from build123d import *

# Parameters (mm, degrees)
SK_PLATE_W              = 160
SK_PLATE_H              = 40
EX_PLATE_DEPTH          = 5
SK_PADPOCKETS_W         = 26
SK_PADPOCKETS_H         = 20
CUT_PADPOCKETS_DEPTH    = 1
SK_PADINSERTS_M3_R      = 2
CUT_PADINSERTS_M3_DEPTH = 5
SK_MAGNET_R             = 3
CUT_MAGNET_DEPTH        = 3
SK_FRAMEBOLTS_R         = 2.15
CUT_FRAMEBOLTS_DEPTH    = 5


with BuildPart() as part:
    # SK_Plate → EX_Plate (new body)
    with BuildSketch(Plane(origin=(0, 0, 0), x_dir=(1, 0, 0), z_dir=(0, 1, 0))):
        Rectangle(SK_PLATE_W, SK_PLATE_H)
    extrude(amount=EX_PLATE_DEPTH)

    # SK_PadPockets → CUT_PadPockets (cut)
    with BuildSketch(Plane(origin=(0, 0, 0), x_dir=(1, 0, 0), z_dir=(0, 1, 0))):
        with Locations((64, 0)):
            Rectangle(SK_PADPOCKETS_W, SK_PADPOCKETS_H)
        with Locations((-64, 0)):
            Rectangle(SK_PADPOCKETS_W, SK_PADPOCKETS_H)
    extrude(amount=CUT_PADPOCKETS_DEPTH, mode=Mode.SUBTRACT)

    # SK_PadInserts_M3 → CUT_PadInserts_M3 (cut)
    with BuildSketch(Plane(origin=(0, 0, 0), x_dir=(1, 0, 0), z_dir=(0, 1, 0))):
        with Locations(Location((64, 0, 0), (0, 0, 270))):
            Circle(SK_PADINSERTS_M3_R)
        with Locations(Location((-64, 0, 0), (0, 0, 270))):
            Circle(SK_PADINSERTS_M3_R)
    extrude(amount=CUT_PADINSERTS_M3_DEPTH, mode=Mode.SUBTRACT)

    # SK_Magnet → CUT_Magnet (cut)
    with BuildSketch(Plane(origin=(0, 0, 0), x_dir=(1, 0, 0), z_dir=(0, 1, 0))):
        with Locations(Location((0, 0, 0), (0, 0, 270))):
            Circle(SK_MAGNET_R)
    extrude(amount=CUT_MAGNET_DEPTH, mode=Mode.SUBTRACT)

    # SK_FrameBolts → CUT_FrameBolts (cut)
    with BuildSketch(Plane(origin=(0, 0, 0), x_dir=(1, 0, 0), z_dir=(0, 1, 0))):
        with Locations(Location((60, 14, 0), (0, 0, 270))):
            Circle(SK_FRAMEBOLTS_R)
        with Locations(Location((-60, 14, 0), (0, 0, 270))):
            Circle(SK_FRAMEBOLTS_R)
    extrude(amount=CUT_FRAMEBOLTS_DEPTH, mode=Mode.SUBTRACT)


solid = part.part
Work out the finished part from the listing and answer in its coordinate system (mm). A direction names the side the tool comes from. Coordinates: 2 decimals unless noted, no trailing zeros. Loops run counter-clockwise (first coordinate to the right, second up) from the corner with the lowest first, then second, coordinate; pieces in that order, holes last. Notation, with made-up numbers: M 0.5,-3.75 L 9.5,-3.75 A26 cw 9.5,11.25 Z; hole C 25.5,80 d11. An arc over 180 degrees is marked long. Answer in a Markdown table with one row per item. Add a question column.
1. Flat-ended cylindrical pins translate along their axes: P1, Ø5, axis at x = 64, z = 0, coming from the +Y side; P2, Ø6, axis at x = 69.5, z = -4.5, coming from the -Y side. Find the tip coordinate at first contact, or state that the pin passes through.
2. A tool of negligible diameter and unlimited length cuts with its end or side. For faces 1 (the flat face through (-64.2, 1, -2.4)), 2 (the cylindrical face through (65.686, 2.972, 1.075)), from which of +Z, -Z, +X, -X, +Y, -Y can it reach the whole face along a straight path? Write none if from no direction.
3. Consider L1, parallel to X at y = 1.45, z = -14; L2, parallel to X at y = 0.95, z = 5; L3, parallel to X at y = 1.45, z = 0. Determine where each line is inside the solid, lowest interval first.
4. Find section C-C, the plane z = -5.5. Write down the section's boundary in (x, y).
5. Find section B-B, the plane x = -64. Write down the section's boundary in (y, z), then the cut area to 3 significant figures.
6. The mould has two halves that part along Z. Classify faces 3 (the cylindrical face through (0.9, 1.48, 2.86)), 4 (the flat face through (0, 3, 0)), 5 (the flat face through (-1, 2, 20)), 6 (the flat face through (-1, 5, 0)): pulls with the +Z half, pulls with the -Z half, needs draft (parallel to the pull), parting line crosses it, or undercut.
7. Find section D-D, the plane x = 60. Write down the section's boundary in (y, z), then the cut area to 4 significant figures.
8. Find section A-A, the plane z = -14. Write down the section's boundary in (x, y).
Reported:
| question | item | result |
|---|---|---|
| 1 | P1 | stops at y = 5 |
| 1 | P2 | stops at y = 1 |
| 2 | face 1 | -Y |
| 2 | face 2 | +Y, -Y |
| 3 | L1 | x = -80 to -62.15, -57.85 to 57.85, 62.15 to 80 |
| 3 | L2 | x = -80 to -77, -51 to 51, 77 to 80 |
| 3 | L3 | x = -80 to -66, -62 to -3, 3 to 62, 66 to 80 |
| 4 | outline | M -80,0 L -77,0 L -77,1 L -51,1 L -51,0 L 51,0 L 51,1 L 77,1 L 77,0 L 80,0 L 80,5 L -80,5 Z |
| 5 | outline | M 0,-20 L 5,-20 L 5,-2 L 1,-2 L 1,-10 L 0,-10 Z; M 0,10 L 1,10 L 1,2 L 5,2 L 5,20 L 0,20 Z |
| 5 | area | 164 mm^2 |
| 6 | face 3 | undercut |
| 6 | face 4 | undercut |
| 6 | face 5 | pulls with the +Z half |
| 6 | face 6 | needs draft |
| 7 | outline | M 0,-20 L 5,-20 L 5,-16.15 L 0,-16.15 Z; M 0,-11.85 L 5,-11.85 L 5,20 L 0,20 L 0,10 L 1,10 L 1,-10 L 0,-10 Z |
| 7 | area | 158.5 mm^2 |
| 8 | outline | M -80,0 L -62.15,0 L -62.15,5 L -80,5 Z; M -57.85,0 L 57.85,0 L 57.85,5 L -57.85,5 Z; M 62.15,0 L 80,0 L 80,5 L 62.15,5 Z |
